```python
from build123d import *

# Parameters (mm, degrees)
SKETCH1_W     = 50
SKETCH1_H     = 50
SKETCH1_R     = 1.5
SUPPORT_DEPTH = 8


with BuildPart() as part:
    # Sketch1 → Support (new body)
    with BuildSketch(Plane(origin=(0, 0, 0), x_dir=(1, 0, 0), z_dir=(0, 1, 0))):
        Rectangle(SKETCH1_W, SKETCH1_H)
        with Locations(Location((-21, -21, 0), (0, 0, 270))):
            Circle(SKETCH1_R, mode=Mode.SUBTRACT)
        with Locations(Location((21, -21, 0), (0, 0, 270))):
            Circle(SKETCH1_R, mode=Mode.SUBTRACT)
        with BuildLine():
            Line((-13.031373033, 17.5), (17.5, 17.5))
            Line((17.5, 17.5), (17.5, -17.5))
            Line((17.5, -17.5), (-17.5, -17.5))
            Line((-17.5, -17.5), (-17.5, 13.031373033))
            ThreePointArc((-17.5, 13.031373033), (-20, 14.354248689), (-21, 17))
            Line((-21, 17), (-22.130136986, 20.01369863))
            ThreePointArc((-22.130136986, 20.01369863), (-22.060660172, 22.060660172), (-20.01369863, 22.130136986))
            Line((-20.01369863, 22.130136986), (-17, 21))
            ThreePointArc((-17, 21), (-14.354248689, 20), (-13.031373033, 17.5))
        make_face(mode=Mode.SUBTRACT)
        with Locations(Location((21, 21, 0), (0, 0, 270))):
            Circle(SKETCH1_R, mode=Mode.SUBTRACT)
    extrude(amount=SUPPORT_DEPTH)


solid = part.part
```
Check sheet for the modelled part. Datum: model origin and axes. Units: mm. A direction names the side the tool comes from. Coordinates: 2 decimals unless noted, no trailing zeros. Loops run counter-clockwise (first coordinate to the right, second up) from the corner with the lowest first, then second, coordinate; pieces in that order, holes last.
1) Material ranges on probe 1 along X at (y, z) = (5.75, 21); probe 2 along Z at (x, y) = (8, 4.5), recorded low to high.
2) Sectioned sample at B-B (y = 6.5). Record the boundary of the cut face in (x, z).
3) Sectioned sample at C-C (x = 21). Record the boundary of the cut face in (y, z).
4) Access from +Z, -Z, +X, -X, +Y, -Y to the whole of each face (thin tool, end or side, straight path). Record for faces 1 (the face through (0, 4, -25)), 2 (the face through (-17.5, 4, 2)).
5) Sectioned sample at D-D (x = 13.5). Record the boundary of the cut face in (y, z), and give its area (3 significant figures).
6) Release check for a two-part mould opening along Z. For faces 3 (the face through (25, 4, 0)), 4 (the face through (-19.99, 3.94, 19.89)), 5 (the face through (0, 4, 25)) record: released by +Z, released by -Z, zero draft, split by the parting line, or undercut.
7) Sectioned sample at A-A (z = 21). Record the boundary of the cut face in (x, y).
8) Gauge pin test, flat end, axial feed: pin 1 (1.8 mm diameter, centred on x = 21, z = 21, fed in from -Y). Record the tip position at first contact, or that the pin passes through.
Check sheet entries:
1. probe 1: x = -25 to -22.5, -19.5 to 19.5, 22.5 to 25
1. probe 2: z = -25 to -17.5, 17.5 to 25
2. outline: (-25, -25) - (25, -25) - (25, 25) - (-25, 25) - close; hole circle Ø3 at (-21, 21); hole (-22.13, -20.01) arc R1.5 ccw to (-20.01, -22.13) - (-17, -21) arc R4 ccw to (-13.03, -17.5) - (17.5, -17.5) - (17.5, 17.5) - (-17.5, 17.5) - (-17.5, -13.03) arc R4 ccw to (-21, -17) - close; hole circle Ø3 at (21, -21); hole circle Ø3 at (21, 21)
3. outline: (0, -25) - (8, -25) - (8, -22.5) - (0, -22.5) - close; (0, -19.5) - (8, -19.5) - (8, 19.5) - (0, 19.5) - close; (0, 22.5) - (8, 22.5) - (8, 25) - (0, 25) - close
4. face 1: -Z, +X, -X, +Y, -Y
4. face 2: +Y, -Y
5. outline: (0, -25) - (8, -25) - (8, -17.5) - (0, -17.5) - close; (0, 17.5) - (8, 17.5) - (8, 25) - (0, 25) - close
5. area: 120 mm2
6. face 3: zero draft
6. face 4: undercut
6. face 5: released by +Z
7. outline: (-25, 0) - (-22.5, 0) - (-22.5, 8) - (-25, 8) - close; (-19.5, 0) - (19.5, 0) - (19.5, 8) - (-19.5, 8) - close; (22.5, 0) - (25, 0) - (25, 8) - (22.5, 8) - close
8. pin 1: passes through
